The listing builds one solid part. Answer for the finished solid, in the listing's coordinates (mm). A direction names the side the tool comes from. Round coordinates to 2 decimals unless told otherwise and drop trailing zeros. Order: outer loops, then holes, each group sorted by start corner. A loop starts at its lowest first (then second) coordinate and runs counter-clockwise, first axis right, second up. Notation, with made-up numbers: (40.25, 15.25) - (63.25, 15.25) arc R16 cw to (63.25, 20.25) - close; hole circle Ø7 at (-10, -26). An arc over 180 degrees is marked (long way). Use CSV: the item, a comma, the result in double quotes. Start each with the question number.
Item 1: Flat-ended cylindrical pins translate along their axes: P1, Ø1, axis at y = 15, z = 4, coming from the -X side; P2, Ø6, axis at y = 16.5, z = 10.5, coming from the -X side; P3, Ø6.5, axis at x = 0, y = 10, coming from the +Z side. Find the tip coordinate at first contact, or state that the pin passes through.
Item 2: Find section B-B, the plane y = 10. Give the vertices of the cut face in (x, z).
Item 3: Straight lines are drawn through the part: line 1 along Y through (x, z) = (0, 2.5); line 2 along Z through (x, y) = (13.5, 13.5); line 3 along X through (y, z) = (3, 6.5). For each, find the intervals that lie inside material, in ascending order. Write a range as [from, to].
Item 4: Find section A-A, the plane x = 0. Give the vertices of the cut face in (y, z), plus the area to 3 significant figures.
Item 5: For faces 3 (the flat face through (0.2, 7.6, 7.11)), 4 (the cylindrical face through (30.62, 9.86, 7.5)), determine the directions among +Z, -Z, +X, -X, +Y, -Y from which every point of the face is accessible in a straight line to the end or side of a thin tool.
Item 6: Determine the mould class of faces 1 (the flat face through (1, 20, 5)), 2 (the cylindrical face through (29.715, 9.86, 11.864)) for opening direction X: +X half, -X half, draft (parallel to the pull), parting line (faces both ways), or undercut.
Item 7: Find section C-C, the plane z = 2.25. Give the vertices of the cut face in (x, y).
Item 8: Find section D-D, the plane z = 11.75. Give the vertices of the cut face in (x, y).
```python
from build123d import *

# Parameters (mm, degrees)
BOSS_EXTRUDE1_DEPTH = 20
SKETCH2_R           = 2.01
CUT_EXTRUDE1_DEPTH  = 20


with BuildPart() as part:
    # Sketch1 → Boss-Extrude1 (new body)
    with BuildSketch(Plane(origin=(0, 0, 0), x_dir=(1, 0, 0), z_dir=(0, 1, 0))):
        with BuildLine():
            Line((-23.28, 0), (23.28, 0))
            ThreePointArc((23.28, 0), (30.78, -7.5), (38.28, 0))
            ThreePointArc((38.28, 0), (29.504120366, -11.932347946), (15.4990516, -7.11))
            Line((15.4990516, -7.11), (-15.4990516, -7.11))
            ThreePointArc((-15.4990516, -7.11), (-29.504120366, -11.932347946), (-38.28, 0))
            ThreePointArc((-38.28, 0), (-30.78, -7.5), (-23.28, 0))
        make_face()
    extrude(amount=BOSS_EXTRUDE1_DEPTH)

    # Sketch2 → Cut-Extrude1 (cut)
    with BuildSketch(Plane(origin=(0, 0, 0), x_dir=(-1, 0, 0), z_dir=(0, 0, -1))):
        with Locations((0, 10)):
            Circle(SKETCH2_R)
    extrude(amount=-CUT_EXTRUDE1_DEPTH, mode=Mode.SUBTRACT)


solid = part.part
```
Worked out:
1,P1,"stops at x = -37.78"
1,P2,"stops at x = -35.78"
1,P3,"stops at z = 7.11"
2,outline,"(-38.28, 0) arc R7.5 cw to (-23.28, 0) - (-2.01, 0) - (-2.01, 7.11) - (-15.5, 7.11) arc R12.5 ccw to start; (2.01, 0) - (23.28, 0) arc R7.5 cw to (38.28, 0) arc R12.5 ccw to (15.5, 7.11) - (2.01, 7.11) - close"
3,line 1,"y = [0, 7.99], [12.01, 20]"
3,line 2,"z = [0, 7.11]"
3,line 3,"x = [-36.46, -34.52], [-27.04, 27.04], [34.52, 36.46]"
4,outline,"(0, 0) - (7.99, 0) - (7.99, 7.11) - (0, 7.11) - close; (12.01, 0) - (20, 0) - (20, 7.11) - (12.01, 7.11) - close"
4,area,"114 mm²"
5,face 3,"+Z, +Y, -Y"
5,face 4,"-Z, +Y, -Y"
6,face 1,"draft"
6,face 2,"undercut"
7,outline,"(-38.08, 0) - (-37.93, 0) - (-37.93, 20) - (-38.08, 20) - close; (-23.63, 0) - (23.63, 0) - (23.63, 20) - (-23.63, 20) - close; (37.93, 0) - (38.08, 0) - (38.08, 20) - (37.93, 20) - close; hole circle Ø4.02 at (0, 10)"
8,outline,"(-30.04, 0) - (-21.52, 0) - (-21.52, 20) - (-30.04, 20) - close; (21.52, 0) - (30.04, 0) - (30.04, 20) - (21.52, 20) - close"
